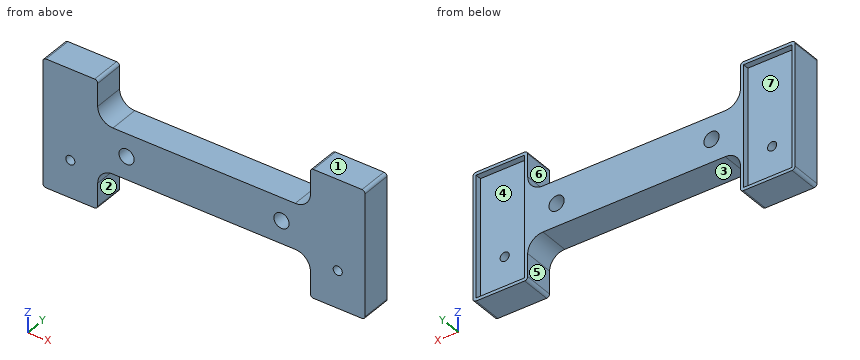
```python
from build123d import *

# Parameters (mm, degrees)
SKETCH1_W           = 70
SKETCH1_H           = 15
SKETCH1_R           = 2.5
BOSS_EXTRUDE2_DEPTH = 10
FILLET1_R           = 5
SKETCH4_W           = 16
SKETCH4_H           = 40
CUT_EXTRUDE2_DEPTH  = 2
SKETCH5_R           = 1.5
CUT_EXTRUDE3_DEPTH  = 58.567351858
FILLET2_R           = 1


with BuildPart() as part:
    # Sketch1 → Boss-Extrude2 (new body)
    # profile 1 of 3: a face of its own
    with BuildSketch(Plane(origin=(0, 0, 0), x_dir=(1, 0, 0), z_dir=(0, 1, 0))):
        Polygon((-35, -7.5), (-35, 7.5), (-35, 21), (-53, 21), (-53, -21), (-35, -21), align=None)
    # profile 2 of 3: a face of its own
    with BuildSketch(Plane(origin=(0, 0, 0), x_dir=(1, 0, 0), z_dir=(0, 1, 0))):
        Rectangle(SKETCH1_W, SKETCH1_H)
        with Locations(Location((25.5, 0, 0), (0, 0, 270))):
            Circle(SKETCH1_R, mode=Mode.SUBTRACT)
        with Locations(Location((-25.5, 0, 0), (0, 0, 270))):
            Circle(SKETCH1_R, mode=Mode.SUBTRACT)
    # profile 3 of 3: a face of its own
    with BuildSketch(Plane(origin=(0, 0, 0), x_dir=(1, 0, 0), z_dir=(0, 1, 0))):
        Polygon((35, 21), (35, 7.5), (35, -7.5), (35, -21), (53, -21), (53, 21), align=None)
    extrude(amount=BOSS_EXTRUDE2_DEPTH)

    # Fillet1
    fillet1_edges = [part.edges().sort_by_distance(p)[0] for p in [
        (-35, 5, -7.5),
        (35, 5, -7.5),
        (35, 5, 7.5),
        (-35, 5, 7.5),
    ]]
    fillet(fillet1_edges, radius=FILLET1_R)

    # Sketch4 → Cut-Extrude2 (cut)
    with BuildSketch(Plane(origin=(0, 10, 0), x_dir=(1, 0, 0), z_dir=(0, 1, 0))):
        with Locations((-44, 0)):
            Rectangle(SKETCH4_W, SKETCH4_H)
    cut_extrude2 = extrude(amount=-CUT_EXTRUDE2_DEPTH, mode=Mode.SUBTRACT)

    # Mirror3: Cut-Extrude2 across plane
    add(cut_extrude2.mirror(Plane(origin=(0, 0, 0), x_dir=(0, 0, 1), z_dir=(1, 0, 0))), mode=Mode.SUBTRACT)

    # Sketch5 → Cut-Extrude3 (cut, symmetric)
    with BuildSketch(Plane(origin=(0, 8, 0), x_dir=(1, 0, 0), z_dir=(0, 1, 0))):
        with Locations(Location((44, 8.71, 0), (0, 0, 270))):
            Circle(SKETCH5_R)
    cut_extrude3 = extrude(amount=CUT_EXTRUDE3_DEPTH, both=True, mode=Mode.SUBTRACT)

    # Mirror4: Cut-Extrude3 across plane
    add(cut_extrude3.mirror(Plane(origin=(0, 0, 0), x_dir=(0, 0, 1), z_dir=(1, 0, 0))), mode=Mode.SUBTRACT)

    # Fillet2
    fillet2_edges = [part.edges().sort_by_distance(p)[0] for p in [
        (35, 5, -21),
        (53, 5, -21),
        (53, 5, 21),
        (35, 5, 21),
        (-35, 5, 21),
        (-53, 5, 21),
        (-53, 5, -21),
        (-35, 5, -21),
    ]]
    fillet(fillet2_edges, radius=FILLET2_R)


solid = part.part
```
Check sheet for the modelled part. Datum: model origin and axes. Units: mm. Face numbers are marked on the shaded views. A direction names the side the tool comes from. Give positions to 0.01 mm unless a question says otherwise; leave off trailing zeros. Loops run counter-clockwise (first coordinate to the right, second up) from the corner with the lowest first, then second, coordinate; pieces in that order, holes last. Notation, with made-up numbers: M -23.5,56 L 16.5,56 A19 ccw 16.5,83 Z; hole C 80,46.5 d1. An arc over 180 degrees is marked long. Answer in a Markdown table with one row per item.
1) Cross-section at C-C (x = -25.5). Enter the section's corners in (y, z), plus the area to 3 significant figures.
Solutions:
| item | result |
|---|---|
| outline | M 0,-7.5 L 10,-7.5 L 10,-2.5 L 0,-2.5 Z; M 0,2.5 L 10,2.5 L 10,7.5 L 0,7.5 Z |
| area | 100 mm^2 |
2) Tool access check on the marked faces 5, 6 and 7. Record the directions out of +Z, -Z, +X, -X, +Y, -Y that give a thin tool (end or side, any length) a straight path to the whole face; none if there is none.
Solutions:
| item | result |
|---|---|
| face 5 | -Z, +Y, -Y |
| face 6 | +Z, +Y, -Y |
| face 7 | +Y |
3) Cross-section at D-D (y = 5). Enter the section's corners in (x, z), plus the area to 3 significant figures.
Solutions:
| item | result |
|---|---|
| outline | M -53,-20 A1 ccw -52,-21 L -36,-21 A1 ccw -35,-20 L -35,-12.5 A5 cw -30,-7.5 L 30,-7.5 A5 cw 35,-12.5 L 35,-20 A1 ccw 36,-21 L 52,-21 A1 ccw 53,-20 L 53,20 A1 ccw 52,21 L 36,21 A1 ccw 35,20 L 35,12.5 A5 cw 30,7.5 L -30,7.5 A5 cw -35,12.5 L -35,20 A1 ccw -36,21 L -52,21 A1 ccw -53,20 Z; hole C -44,-8.71 d3; hole C -25.5,0 d5; hole C 25.5,0 d5; hole C 44,-8.71 d3 |
| area | 2,530 mm^2 |
4) Cross-section at A-A (z = 0). Enter the section's corners in (x, y).
Solutions:
| item | result |
|---|---|
| outline | M -53,0 L -28,0 L -28,10 L -36,10 L -36,8 L -52,8 L -52,10 L -53,10 Z; M -23,0 L 23,0 L 23,10 L -23,10 Z; M 28,0 L 53,0 L 53,10 L 52,10 L 52,8 L 36,8 L 36,10 L 28,10 Z |
5) Mould release check, pull along Z, two halves, no side actions. Record for the marked faces 1, 2, 3 and 4: released by +Z, released by -Z, zero draft, split by the parting line, or undercut.
Solutions:
| item | result |
|---|---|
| face 1 | released by +Z |
| face 2 | zero draft |
| face 3 | released by -Z |
| face 4 | undercut |
6) Cross-section at B-B (z = -14.5). Enter the section's corners in (x, y).
Solutions:
| item | result |
|---|---|
| outline | M -53,0 L -35,0 L -35,10 L -36,10 L -36,8 L -52,8 L -52,10 L -53,10 Z; M 35,0 L 53,0 L 53,10 L 52,10 L 52,8 L 36,8 L 36,10 L 35,10 Z |
7) Thickness scan on line 1 (X direction, y = 7, z = 0); line 2 (X direction, y = 9.5, z = 17.5); line 3 (X direction, y = 6.25, z = -8.71). Record the ranges inside material, lowest first.
Solutions:
| item | result |
|---|---|
| line 1 | x = -53 to -28, -23 to 23, 28 to 53 |
| line 2 | x = -53 to -52, -36 to -35, 35 to 36, 52 to 53 |
| line 3 | x = -53 to -45.5, -42.5 to -33.26, 33.26 to 42.5, 45.5 to 53 |
8) Depth check by flat-ended pin: pin 1 (12 mm diameter, centred on x = -33, z = -11.5, fed in from -Y); pin 2 (1.8 mm diameter, centred on x = 44, z = -8.71, fed in from -Y); pin 3 (1 mm diameter, centred on x = -23.5, y = 7, fed in from -Z). Enter the tip coordinate at first touch or a pass-through.
Solutions:
| item | result |
|---|---|
| pin 1 | stops at y = 0 |
| pin 2 | passes through |
| pin 3 | stops at z = -7.5 |
